Geometry check sheet. Reference: drawing and pictorial views, mm from the part's lowest x, y, z. A direction names the side the tool comes from. Coordinates: 2 decimals unless noted, no trailing zeros. Loops run counter-clockwise (first coordinate to the right, second up) from the corner with the lowest first, then second, coordinate; pieces in that order, holes last. Notation, with made-up numbers: (-9, 83) -> (24, 83) arc R11 cw to (24, 94) -> close; hole circle Ø1 at (34, 88.5). An arc over 180 degrees is marked (long way). Answer as a JSON object with one key per item and string values. Group by question number.
Q1. Set-up check for the marked faces 1 and 2: record each of +Z, -Z, +X, -X, +Y, -Y from which the full face is reachable in a straight line by a thin tool's end or side.
Q2. Scan lines: L1, parallel to Z at x = 0.3, y = 2.3; L2, parallel to Z at x = 3.35, y = 2.75; L3, parallel to X at y = 2.55, z = 11.25. Record each from-to range of solid material in increasing order.
Q3. Gauge pin test, flat ends, axial feed: pin 1 Ø0.9 at (x, z) = (1.5, 0.5) entering from +Y; pin 2 Ø0.6 at (x, z) = (4, 0.5) entering from +Y; pin 3 Ø0.6 at (x, z) = (4, 0) entering from -Y (1 decimal). Record the tip position at first contact, or that the pin passes through.
Q4. Cross-section at A-A on z = 14.5. Record the boundary of the cut face in (x, y).
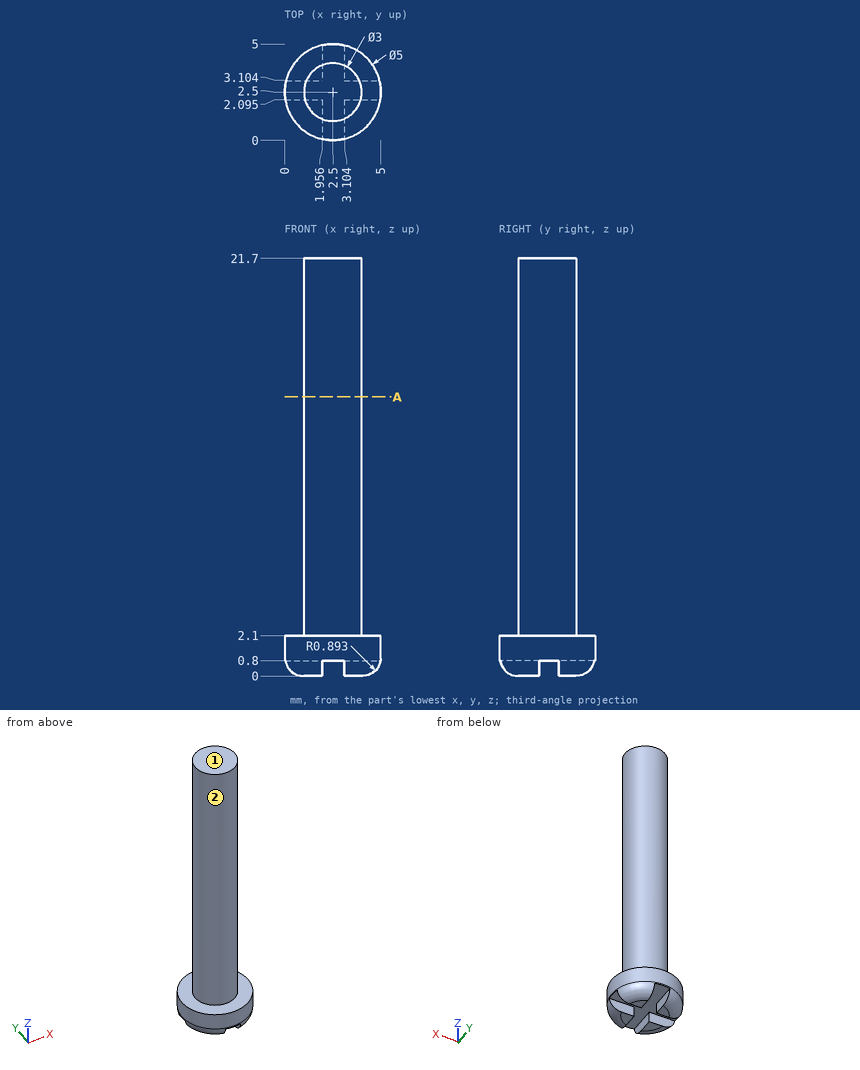
Computed values:
{
 "1": {"face 1": "+Z, +X, -X, +Y, -Y", "face 2": "+Z"},
 "2": {"L1": "z = 0.8 to 2.1", "L2": "z = 0.8 to 21.7", "L3": "x = 1 to 4"},
 "3": {"pin 1": "stops at y = 4.91", "pin 2": "stops at y = 4.63", "pin 3": "stops at y = 0.7"},
 "4": {"outline": "circle Ø3 at (2.5, 2.5)"}
}
